For this review, take the finished solid that the model builds, in its own axes (mm). A direction names the side the tool comes from. Coordinates: 2 decimals unless noted, no trailing zeros. Write each loop counter-clockwise with the first axis right and the second up, starting at its lowest first coordinate (ties: lowest second). Pieces come first, ordered by that corner, then holes.
1) Mouldability with a two-part tool opening along Z and no side actions: class faces 6 (the face through (0, -11, -8.4)), 7 (the face through (-2, -2, -5.6)), 8 (the face through (-2, 9, 9.6)), 9 (the face through (9.79, -4.06, -0.12)) as pulls with the +Z half, pulls with the -Z half, needs draft (parallel to the pull), parting line crosses it, or undercut.
2) To check wall thickness, follow line 1 along Y through (x, z) = (0, -6.9); line 2 along Y through (x, z) = (0, 7.35). State the ranges of each line that lie inside material, in increasing order.
3) We need section C-C on z = 4.75. Write out the cut boundary in (x, y).
4) Insertion check: P1, Ø6, axis at y = 4, z = 6.5, coming from the -X side; P2, Ø3, axis at y = -2, z = -2.5, coming from the +X side; P3, Ø5, axis at y = -6.5, z = -4, coming from the -X side. Each pin has a flat end and moves straight along its axis. Give the tip position at first contact, or say it passes through.
5) We need section A-A on x = -9.5. Write out the cut boundary in (y, z).
6) We need section B-B on z = -6.75. Write out the cut boundary in (x, y).
7) For faces 1 (the face through (1.107, -8.428, 7.832)), 2 (the face through (0, -11, 8.4)), 3 (the face through (0.534, 4.065, -7.374)), 4 (the face through (11.18, -4.63, 8.99)), 5 (the face through (0, -5, -9.6)), list the 3-axis set-ups (+Z, -Z, +X, -X, +Y, -Y) from which the entire face can be reached by the end or side of a thin tool; tool diameter is ignored.
from build123d import *
from OCP.BRepFilletAPI import BRepFilletAPI_MakeChamfer

# Parameters (mm, degrees)
LAUFRAD_DEPTH             = 8.4
LAUFRAD_DEPTH_BACK        = 8.4
SKIZZE1_R                 = 10.6
SKIZZE2_R                 = 12.1
KETTENF_HRUNG_DEPTH       = 1.2
SKIZZE4_R                 = 1.65
SCHRAUBENBOHRUNG_M3_DEPTH = 26.718864672
SKIZZE3_R                 = 4.1
KUGELLAGERSITZ_DEPTH      = 4
FASE1_SIZE                = 0.5
FASE1_SIZE2               = 0.71146453


with BuildPart() as part:
    # Skizze1 → Laufrad (new, two sides: drawn at the far end of the back side and taken through both)
    with BuildSketch(Plane.XY.offset(-LAUFRAD_DEPTH_BACK)):
        Circle(SKIZZE1_R)
    extrude(amount=LAUFRAD_DEPTH + LAUFRAD_DEPTH_BACK)

    # Skizze2 → Kettenf_hrung (add)
    with BuildSketch(Plane.XY.offset(8.4)):
        Circle(SKIZZE2_R)
    kettenf_hrung = extrude(amount=KETTENF_HRUNG_DEPTH)

    # Spiegeln Kettenf_hrung: Kettenf_hrung across plane
    add(kettenf_hrung.mirror(Plane.XY))

    # Skizze4 → SchraubenBohrung M3 (cut, through all)
    with BuildSketch(Plane(origin=(0, 0, -9.6), x_dir=(-1, 0, 0), z_dir=(0, 0, -1))):
        Circle(SKIZZE4_R)
    extrude(amount=-SCHRAUBENBOHRUNG_M3_DEPTH, mode=Mode.SUBTRACT)

    # Skizze3 → Kugellagersitz (cut)
    with BuildSketch(Plane(origin=(0, 0, -9.6), x_dir=(-1, 0, 0), z_dir=(0, 0, -1))):
        Circle(SKIZZE3_R)
    extrude(amount=-KUGELLAGERSITZ_DEPTH, mode=Mode.SUBTRACT)

    # Skizze5 → Schnitt-Rotation3 (revolve, cut)
    with BuildSketch(Plane(origin=(0, 0, 0), x_dir=(0, 0, -1), z_dir=(1, 0, 0)), mode=Mode.PRIVATE) as schnitt_rotation3_sk:
        Polygon((-9.6, 0), (-9.6, 8.5), (-6.6, 8.5), (2.6, 6), (2.6, 0), align=None)
    revolve(schnitt_rotation3_sk.sketch.rotate(Axis((0, 0, -8.4), (0, 0, 1)), 90), axis=Axis((0, 0, -8.4), (0, 0, 1)), mode=Mode.SUBTRACT)

    # Fase1: one chamfer whose edges measure the first distance from different faces: ONE call of the kernel's chamfer builder (chamfer() names one face for all edges)
    fase1_edges_1 = [part.edges().sort_by_distance(p)[0] for p in [
        (4.1, 0, -9.6),
        (1.65, 0, -5.6),
        (1.65, 0, -2.6),
        (8.5, 0, 9.6),
    ]]
    fase1_edges_2 = [part.edges().sort_by_distance(p)[0] for p in [
        (6, 0, -2.6),
    ]]
    fase1_side_2 = [part.faces().sort_by_distance(p)[0] for p in [
        (5.830294373, 0, -2.6),
    ]]
    fase1 = BRepFilletAPI_MakeChamfer(part.part.solid().wrapped)
    for e in fase1_edges_1:
        fase1.Add(FASE1_SIZE, e.wrapped)
    for e in fase1_edges_2:
        fase1.Add(FASE1_SIZE, FASE1_SIZE2, e.wrapped, fase1_side_2[0].wrapped)  # the first distance lies on this face
    add(Compound.cast(fase1.Shape()), mode=Mode.REPLACE)


solid = part.part
Result:
1. face 6: undercut
1. face 7: pulls with the -Z half
1. face 8: pulls with the +Z half
1. face 9: undercut
2. line 1: y = -10.6 to -4.1, 4.1 to 10.6
2. line 2: y = -10.6 to -8.5, 8.5 to 10.6
3. outline: circle Ø21.2 at (0, 0); hole circle Ø15.99 at (0, 0)
4. P1: stops at x = -11.98
4. P2: stops at x = 10.59
4. P3: stops at x = -9.82
5. outline: (-7.49, -9.6) - (7.49, -9.6) - (7.49, -8.4) - (4.7, -8.4) - (4.7, 8.4) - (7.49, 8.4) - (7.49, 9.6) - (-7.49, 9.6) - (-7.49, 8.4) - (-4.7, 8.4) - (-4.7, -8.4) - (-7.49, -8.4) - close
6. outline: circle Ø21.2 at (0, 0); hole circle Ø8.2 at (0, 0)
7. face 1: +Z
7. face 2: none
7. face 3: -Z
7. face 4: +Z, -Z
7. face 5: -Z, +X, -X, +Y, -Y
